The model under review builds one solid part; all positions refer to its coordinate system, in mm. Give positions to 0.01 mm unless a question says otherwise; leave off trailing zeros. Order: outer loops, then holes, each group sorted by start corner. A loop starts at its lowest first (then second) coordinate and runs counter-clockwise, first axis right, second up. Notation, with made-up numbers: (89.5, 7) - (116.5, 7) arc R19 cw to (116.5, 17) - close; hole circle Ø7 at (74, 60). An arc over 180 degrees is marked (long way). Use CSV: the item, a comma, the result in double quotes. Start each with the question number.
1. Take a section at C-C, the plane x = 11.5. State the section outline as (y, z) points, then the cut area to 3 significant figures.
2. To check wall thickness, follow line 1 (X direction, y = 71, z = 2.35); line 2 (X direction, y = 50, z = 0.8); line 3 (Y direction, x = 20, z = 2.2). State the ranges of each line that lie inside material, in increasing order. Write a range as [from, to].
3. Take a section at A-A, the plane z = 1.5. State the section outline as (x, y) points.
4. Take a section at D-D, the plane y = 39. State the section outline as (x, z) points, then the cut area to 3 significant figures.
5. For pin 1 (0.5 mm diameter, centred on x = 53, z = 2.5, fed in from -Y); pin 2 (0.8 mm diameter, centred on y = 78.5, z = 2.5, fed in from +X), all flat-tipped, find the tip position at first contact; note any pin that passes through.
6. Take a section at B-B, the plane y = 63. State the section outline as (x, z) points.
Autodesk Fusion 360 part; units mm, degrees
sketch "Sketch1" plane through (0, 0, 0) normal (0, 0, 1) x (1, 0, 0)
  line L0 (0, 0) -> (61, 0)
  line L1 (61, 0) -> (61, 84)
  line L2 (61, 84) -> (0, 84)
  line L3 (0, 84) -> (0, 0)
  dimension "d1" = 61
  dimension "d2" = 84
extrude "Extrude1" add sketch "Sketch1" along normal blind 2
sketch "Sketch2" plane through (0, 0, 2) normal (0, 0, 1) x (-1, 0, 0)
  line L0 (0, -84) -> (0, 0)
  line L1 (0, 0) -> (-61, 0)
  line L2 (-61, 0) -> (-61, -84)
  line L3 (-61, -84) -> (0, -84)
  line L4 (-2, -2) -> (-59, -2)
  line L5 (-59, -2) -> (-59, -82)
  line L6 (-59, -82) -> (-2, -82)
  line L7 (-2, -82) -> (-2, -2)
  dimension "d5" = 57
  dimension "d6" = 80
extrude "Extrude2" add sketch "Sketch2" along normal blind 1 contours L4 L5 L6 L7
sketch "Sketch3" plane through (0, 0, 3) normal (0, 0, 1) x (-1, 0, 0)
  line L0 (-2, -82) -> (-2, -2)
  line L1 (-2, -2) -> (-59, -2)
  line L2 (-59, -2) -> (-59, -82)
  line L3 (-59, -82) -> (-2, -82)
  line L4 (-59, -82) -> (-53, -82)
  line L5 (-53, -82) -> (-53, -76)
  line L6 (-53, -76) -> (-59, -76)
  line L7 (-59, -76) -> (-59, -82)
extrude "Extrude3" cut sketch "Sketch3" against normal blind 1 contours L2 L3 L4 L5 L6 L7
sketch "Sketch4" plane through (0, 0, 3) normal (0, 0, 1) x (-1, 0, 0)
  line L0 (-53, -76) -> (-53, -82)
  line L1 (-53, -82) -> (-2, -82)
  line L2 (-2, -82) -> (-2, -2)
  line L3 (-2, -2) -> (-59, -2)
  line L4 (-59, -2) -> (-59, -76)
  line L5 (-59, -76) -> (-53, -76)
  line L6 (-2, -82) -> (-8, -82)
  line L7 (-8, -82) -> (-8, -76)
  line L8 (-8, -76) -> (-2, -76)
  line L9 (-2, -76) -> (-2, -82)
extrude "Extrude4" cut sketch "Sketch4" against normal blind 1 contours L1 L2 L6 L7 L8 L9
sketch "Sketch5" plane through (0, 0, 3) normal (0, 0, 1) x (-1, 0, 0)
  line L0 (-8, -76) -> (-2, -76)
  line L1 (-2, -76) -> (-2, -2)
  line L2 (-2, -2) -> (-59, -2)
  line L3 (-59, -2) -> (-59, -76)
  line L4 (-59, -76) -> (-53, -76)
  line L5 (-53, -76) -> (-53, -82)
  line L6 (-53, -82) -> (-8, -82)
  line L7 (-8, -82) -> (-8, -76)
  line L8 (-2, -2) -> (-8, -2)
  line L9 (-8, -2) -> (-8, -8)
  line L10 (-8, -8) -> (-2, -8)
  line L11 (-2, -8) -> (-2, -2)
extrude "Extrude5" cut sketch "Sketch5" against normal blind 1 contours L1 L2 L8 L9 L10 L11
sketch "Sketch6" plane through (0, 0, 2) normal (0, 0, 1) x (-1, 0, 0)
  line L0 (-8, -82) -> (-53, -82)
  line L1 (-53, -82) -> (-53, -76)
  line L2 (-53, -76) -> (-59, -76)
  line L3 (-59, -76) -> (-59, -2)
  line L4 (-59, -2) -> (-8, -2)
  line L5 (-8, -2) -> (-8, -8)
  line L6 (-8, -8) -> (-2, -8)
  line L7 (-2, -8) -> (-2, -76)
  line L8 (-2, -76) -> (-8, -76)
  line L9 (-8, -76) -> (-8, -82)
  line L10 (0, -84) -> (0, 0)
  line L11 (0, 0) -> (-61, 0)
  line L12 (-61, 0) -> (-61, -84)
  line L13 (-61, -84) -> (0, -84)
  line L14 (-14.5, 0) -> (-45.5, 0)
  line L15 (-45.5, 0) -> (-45.5, -2)
  line L16 (-45.5, -2) -> (-14.5, -2)
  line L17 (-14.5, -2) -> (-14.5, 0)
  dimension "d15" = 31
  dimension "d16" = 2
extrude "Extrude6" add sketch "Sketch6" along normal blind 1 contours L4 L11 L14 L15 L16 L17
sketch "Sketch7" plane through (0, 0, 3) normal (0, 0, 1) x (-1, 0, 0)
  line L0 (-8, -8) -> (-8, -2)
  line L1 (-8, -2) -> (-14.5, -2)
  line L2 (-14.5, -2) -> (-14.5, 0)
  line L3 (-14.5, 0) -> (-45.5, 0)
  line L4 (-45.5, 0) -> (-45.5, -2)
  line L5 (-45.5, -2) -> (-59, -2)
  line L6 (-59, -2) -> (-59, -76)
  line L7 (-59, -76) -> (-53, -76)
  line L8 (-53, -76) -> (-53, -82)
  line L9 (-53, -82) -> (-8, -82)
  line L10 (-8, -82) -> (-8, -76)
  line L11 (-8, -76) -> (-2, -76)
  line L12 (-2, -76) -> (-2, -8)
  line L13 (-2, -8) -> (-8, -8)
  line L14 (-53, -17) -> (-59, -17)
  line L15 (-59, -17) -> (-59, -22)
  line L16 (-59, -22) -> (-53, -22)
  line L17 (-53, -22) -> (-53, -17)
  dimension "d19" = 5
extrude "Extrude7" cut sketch "Sketch7" against normal blind 1 contours L6 L14 L15 L16 L17
sketch "Sketch8" plane through (0, 0, 3) normal (0, 0, 1) x (-1, 0, 0)
  line L0 (-53, -22) -> (-59, -22)
  line L1 (-59, -22) -> (-59, -76)
  line L2 (-59, -76) -> (-53, -76)
  line L3 (-53, -76) -> (-53, -82)
  line L4 (-53, -82) -> (-8, -82)
  line L5 (-8, -82) -> (-8, -76)
  line L6 (-8, -76) -> (-2, -76)
  line L7 (-2, -76) -> (-2, -8)
  line L8 (-2, -8) -> (-8, -8)
  line L9 (-8, -8) -> (-8, -2)
  line L10 (-8, -2) -> (-14.5, -2)
  line L11 (-14.5, -2) -> (-14.5, 0)
  line L12 (-14.5, 0) -> (-45.5, 0)
  line L13 (-45.5, 0) -> (-45.5, -2)
  line L14 (-45.5, -2) -> (-59, -2)
  line L15 (-59, -2) -> (-59, -17)
  line L16 (-59, -17) -> (-53, -17)
  line L17 (-53, -17) -> (-53, -22)
  line L18 (-5, -76) -> (-9, -76)
  line L19 (-9, -76) -> (-9, -46)
  line L20 (-9, -46) -> (-5, -46)
  line L21 (-5, -46) -> (-5, -76)
  dimension "d22" = 4
  dimension "d23" = 30
extrude "Extrude8" cut sketch "Sketch8" against normal blind 4 contours L6 L18 L19 L20 L21
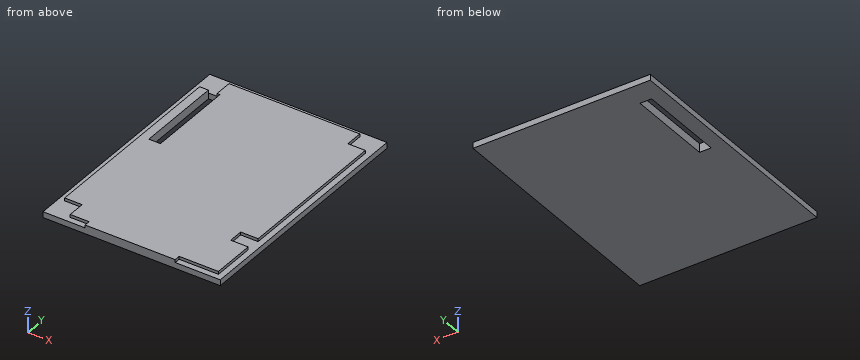
Determined:
1,outline,"(0, 0) - (84, 0) - (84, 2) - (82, 2) - (82, 3) - (2, 3) - (2, 2) - (0, 2) - close"
1,area,"248 mm²"
2,line 1,"x = [2, 5], [9, 59]"
2,line 2,"x = [0, 5], [9, 61]"
2,line 3,"y = [0, 82]"
3,outline,"(0, 0) - (61, 0) - (61, 84) - (0, 84) - close; hole (5, 46) - (9, 46) - (9, 76) - (5, 76) - close"
4,outline,"(0, 0) - (61, 0) - (61, 2) - (59, 2) - (59, 3) - (2, 3) - (2, 2) - (0, 2) - close"
4,area,"179 mm²"
5,pin 1,"stops at y = 2"
5,pin 2,"stops at x = 53"
6,outline,"(0, 0) - (5, 0) - (5, 3) - (2, 3) - (2, 2) - (0, 2) - close; (9, 0) - (61, 0) - (61, 2) - (59, 2) - (59, 3) - (9, 3) - close"
